Could you check a few things on this model? Use its own coordinates, in mm. Face numbers are marked on the shaded views. A direction names the side the tool comes from. Coordinates: 2 decimals unless noted, no trailing zeros. Order: outer loops, then holes, each group sorted by start corner. A loop starts at its lowest first (then second) coordinate and runs counter-clockwise, first axis right, second up. Notation, with made-up numbers: (-26, 75) - (24, 75) arc R22 cw to (24, 109) - close; hole circle Ø2 at (38.25, 59). An arc over 180 degrees is marked (long way). One line per item, written item: value.
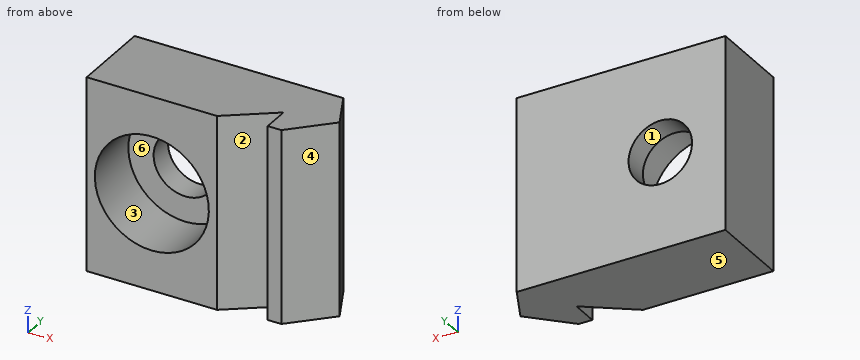
from build123d import *

# Parameters (mm, degrees)
EXTRUDE_1_DEPTH     = 5.95
CUT_EXTRUDE_1_REACH = 17.955
SKETCH_2_R          = 1.95
SKETCH_3_R          = 3.5
CUT_EXTRUDE_2_DEPTH = 3.5


with BuildPart() as part:
    # 스케치1 → 보스-돌출1 (new, symmetric)
    with BuildSketch(Plane.XY):
        Polygon((12.816760605, 0), (0, 0), (0, -5), (8, -5), (10.849275014, -2.899040406), (10.849275014, -4.551199566), (11.683700245, -4.551199566), (13.93379398, -2.290921493), align=None)
    extrude(amount=EXTRUDE_1_DEPTH, both=True)

    # 스케치2 → 컷-돌출1 (cut, up to next)
    with BuildSketch(Plane.XZ.offset(5), mode=Mode.PRIVATE) as cut_extrude_1_sk1:
        with Locations(Location((4, 0, 0), (0, 0, 270))):
            Circle(SKETCH_2_R)
    cut_extrude_1_tool1 = extrude(cut_extrude_1_sk1.sketch, amount=-CUT_EXTRUDE_1_REACH, mode=Mode.PRIVATE) & part.part
    add(cut_extrude_1_tool1.solids().sort_by_distance((4, -5, 0))[0], mode=Mode.SUBTRACT)

    # 스케치3 → 컷-돌출2 (cut)
    with BuildSketch(Plane.XZ.offset(5)):
        with Locations(Location((4, 0, 0), (0, 0, 270))):
            Circle(SKETCH_3_R)
    extrude(amount=-CUT_EXTRUDE_2_DEPTH, mode=Mode.SUBTRACT)


solid = part.part
Item 1: For the marked faces 1, 2 and 3, which set-ups out of +Z, -Z, +X, -X, +Y, -Y let a thin tool reach every point of the face, with its end or its side?
Conclusion:
face 1: +Y, -Y
face 2: +Z, -Z, -Y
face 3: -Y
Item 2: If I drill on probe 1 along X at (y, z) = (-3.5, -1.5); probe 2 along Y at (x, z) = (3.5, -3); probe 3 along Z at (x, y) = (2.75, -3.55), over which ranges is the centre line in solid material (lowest first)?
Conclusion:
probe 1: 0 to 0.84, 7.16 to 10.03, 10.85 to 12.73
probe 2: -1.5 to 0
probe 3: -5.95 to -3.27, 3.27 to 5.95
Item 3: I want a section at D-D on z = -3.75. Please give me the cut outline in (x, y).
Conclusion:
outline: (0, -5) - (8, -5) - (10.85, -2.9) - (10.85, -4.55) - (11.68, -4.55) - (13.93, -2.29) - (12.82, 0) - (0, 0) - close
Item 4: Thinking about a two-plate mould opening in X: for the marked faces 4, 5 and 6, which applies, pulls with the +X half, pulls with the -X half, needs draft (parallel to the pull), parting line crosses it, or undercut?
Conclusion:
face 4: pulls with the +X half
face 5: needs draft
face 6: undercut
Item 5: I'm going to push flat-ended pins straight in: pin 1 Ø2 at (x, z) = (4, 1) entering from -Y; pin 2 Ø0.7 at (x, z) = (11.5, -1) entering from -Y. Where does each tip first touch, or does it pass through?
Conclusion:
pin 1: y = -1.5
pin 2: y = -4.55
Item 6: I want a section at A-A on x = 4. Please give me the cut outline in (y, z), then the cut area to 4 significant figures.
Conclusion:
outline: (-5, -5.95) - (0, -5.95) - (0, -1.95) - (-1.5, -1.95) - (-1.5, -3.5) - (-5, -3.5) - close; (-5, 3.5) - (-1.5, 3.5) - (-1.5, 1.95) - (0, 1.95) - (0, 5.95) - (-5, 5.95) - close
area: 29.15 mm²
Item 7: I want a section at B-B on y = -4. Please give me the cut outline in (x, z).
Conclusion:
outline: (0, -5.95) - (9.36, -5.95) - (9.36, 5.95) - (0, 5.95) - close; (10.85, -5.95) - (12.23, -5.95) - (12.23, 5.95) - (10.85, 5.95) - close; hole circle Ø7 at (4, 0)
Item 8: I want a section at C-C on z = -1.25. Please give me the cut outline in (x, y).
Conclusion:
outline: (0, -5) - (0.73, -5) - (0.73, -1.5) - (2.5, -1.5) - (2.5, 0) - (0, 0) - close; (5.5, -1.5) - (7.27, -1.5) - (7.27, -5) - (8, -5) - (10.85, -2.9) - (10.85, -4.55) - (11.68, -4.55) - (13.93, -2.29) - (12.82, 0) - (5.5, 0) - close
